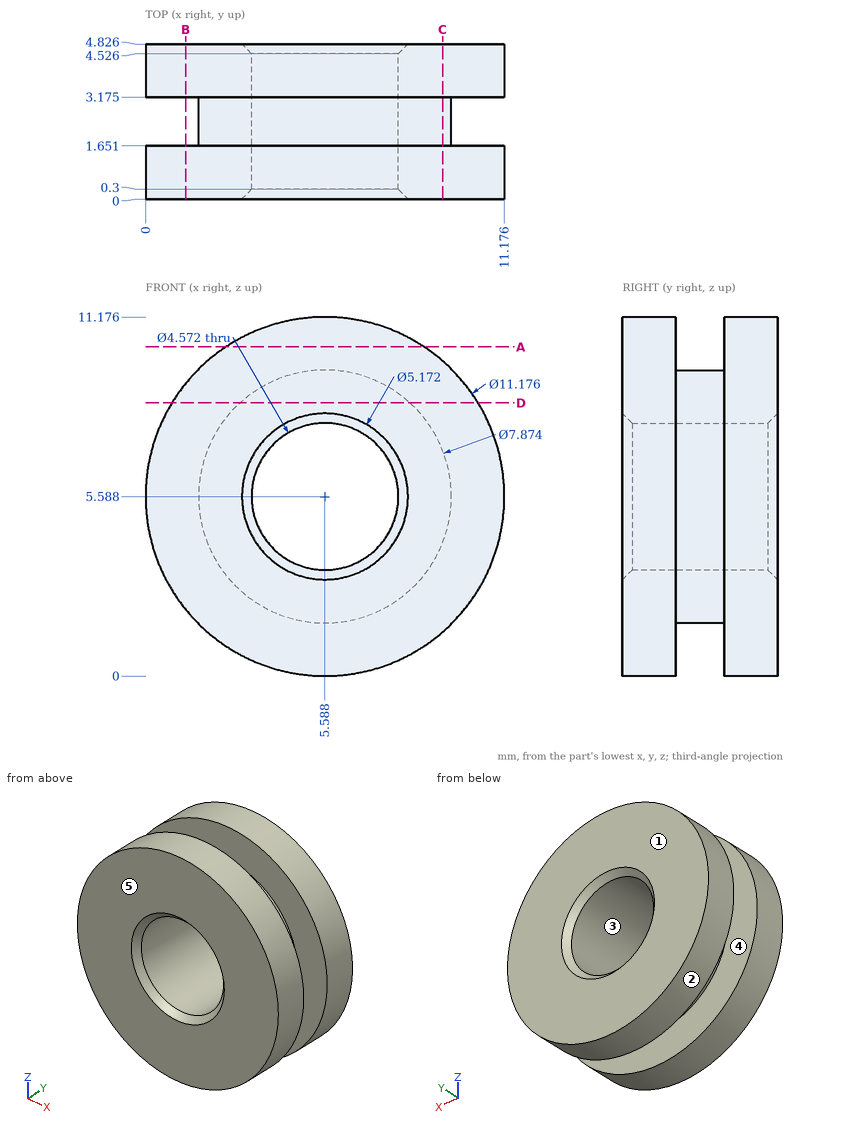
Geometry: see drawing. Coordinates: mm, zero at the bounding-box minimum. A direction names the side the tool comes from. Give positions to 0.01 mm unless a question says otherwise; leave off trailing zeros. Write each loop counter-clockwise with the first axis right and the second up, starting at its lowest first coordinate (ties: lowest second). Pieces come first, ordered by that corner, then holes. Notation, with made-up numbers: M 31.25,71 L 62.25,71 A14 ccw 62.25,95 Z; hole C 17.5,26 d8. An arc over 180 degrees is marked long. Answer in a Markdown table with one row per item. Add a question column.
(1) Section C-C on x = 9.25. Return loops of the section in (y, z) (3 decimals).
(2) Section D-D on z = 8.5. Return loops of the section in (x, y) (3 decimals), and give its area (3 significant figures).
(3) Section B-B on x = 1.25. Return loops of the section in (y, z) (3 decimals).
(4) Mould query, pull axis X, two halves, no side actions, for the marked faces 1, 2 and 3. Classes: +X half, -X half, draft (parallel to the pull), parting line (faces both ways), or undercut.
(5) Section A-A on z = 10.25. Return loops of the section in (x, y) (3 decimals), and give its area (3 significant figures).
(6) Reachability of the marked faces 4 and 5 from +Z, -Z, +X, -X, +Y, -Y: full face, straight path, thin tool, end or side. Return the list, or none.
(7) Ray query, line 1 (Y direction, x = 7.25, z = 1) (3 decimals); line 2 (X direction, y = 2.5, z = 5); line 3 (Z direction, x = 5.75, y = 3.5). Return the intervals inside material, ascending.
(8) First-contact query: pin 1 (2.5 mm diameter, centred on x = 5.588, z = 5.588, fed in from +Y). Flat tip, straight axial feed; report the tip coordinate or a pass-through.
Result set:
| question | item | result |
|---|---|---|
| 1 | outline | M 0,1.367 L 1.651,1.367 L 1.651,4.142 L 3.175,4.142 L 3.175,1.367 L 4.826,1.367 L 4.826,9.809 L 3.175,9.809 L 3.175,7.034 L 1.651,7.034 L 1.651,9.809 L 0,9.809 Z |
| 2 | outline | M 0.819,0 L 10.357,0 L 10.357,1.651 L 8.238,1.651 L 8.238,3.175 L 10.357,3.175 L 10.357,4.826 L 0.819,4.826 L 0.819,3.175 L 2.938,3.175 L 2.938,1.651 L 0.819,1.651 Z |
| 2 | area | 39.6 mm^2 |
| 3 | outline | M 0,2.066 L 1.651,2.066 L 1.651,9.11 L 0,9.11 Z; M 3.175,2.066 L 4.826,2.066 L 4.826,9.11 L 3.175,9.11 Z |
| 4 | face 1 | draft |
| 4 | face 2 | parting line |
| 4 | face 3 | undercut |
| 5 | outline | M 2.507,0 L 8.669,0 L 8.669,1.651 L 2.507,1.651 Z; M 2.507,3.175 L 8.669,3.175 L 8.669,4.826 L 2.507,4.826 Z |
| 5 | area | 20.3 mm^2 |
| 6 | face 4 | none |
| 6 | face 5 | +Z, -Z, +X, -X, -Y |
| 7 | line 1 | y = 0 to 1.651, 3.175 to 4.826 |
| 7 | line 2 | x = 1.7 to 3.38, 7.8 to 9.48 |
| 7 | line 3 | z = 0 to 3.31, 7.87 to 11.17 |
| 8 | pin 1 | passes through |
